Job drawing, mm, ordinate dimensions from the low corner. One solid piece. Give positions to 0.01 mm unless a question says otherwise; leave off trailing zeros. Order: outer loops, then holes, each group sorted by start corner. A loop starts at its lowest first (then second) coordinate and runs counter-clockwise, first axis right, second up.
1. Probe line 1 (Y direction, x = 166.5, z = 1.25); line 2 (Y direction, x = 101, z = 1.75); line 3 (X direction, y = 119, z = 0.35). List the from-to ranges inside material, lowest first.
2. Slice it at A-A on x = 74.5. List the corners of the cut face in (y, z).
3. Slice it at C-C on z = 3.4. Give the number of separate pieces and of enclosed holes in the cut face, and give its area (3 significant figures).
4. Slice it at B-B on y = 65.5. List the corners of the cut face in (x, z), and give its area (3 significant figures).
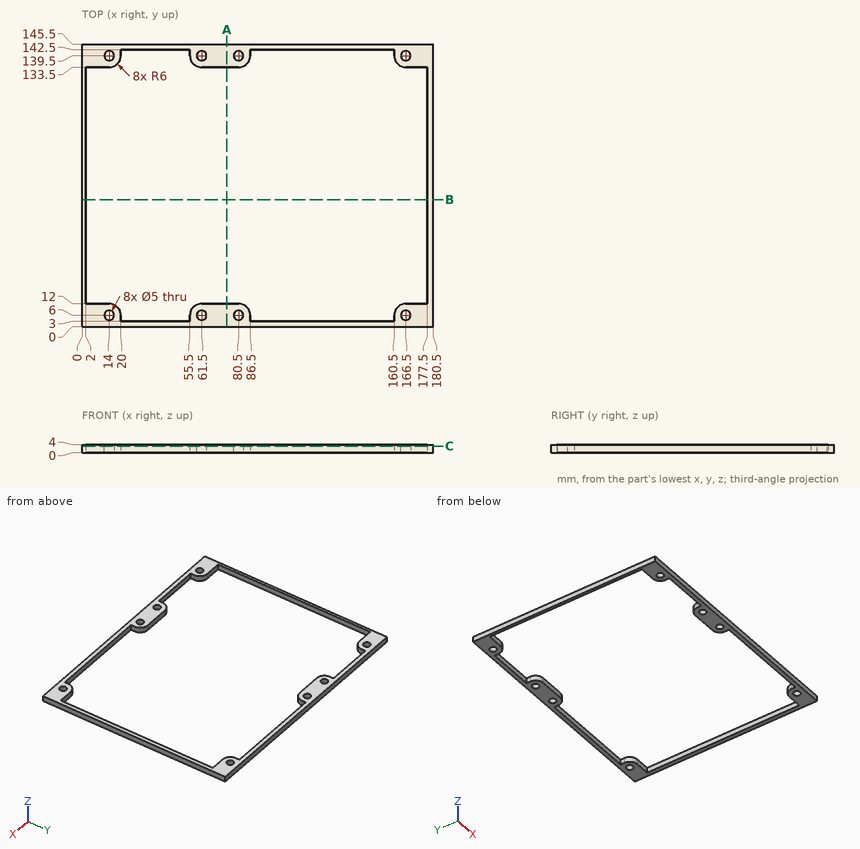
Data:
1. line 1: y = 0 to 3.5, 8.5 to 12, 133.5 to 137, 142 to 145.5
1. line 2: y = 0 to 3, 142.5 to 145.5
1. line 3: x = 0 to 2, 177.5 to 180.5
2. outline: (0, 0) - (12, 0) - (12, 4) - (0, 4) - close; (133.5, 0) - (145.5, 0) - (145.5, 4) - (133.5, 4) - close
3. separate pieces: 1
3. enclosed holes: 9
3. area: 2,750 mm2
4. outline: (0, 0) - (2, 0) - (2, 4) - (0, 4) - close; (177.5, 0) - (180.5, 0) - (180.5, 4) - (177.5, 4) - close
4. area: 20.0 mm2
